from build123d import *

# Parameters (mm, degrees)
SKETCH1_W           = 6
SKETCH1_H           = 10
BOSS_EXTRUDE1_DEPTH = 8
FILLET2_RADIUS      = 3
FILLET2_LENGTH      = 10
SKETCH2_R           = 1.5
BOSS_EXTRUDE2_DEPTH = 2


with BuildPart() as part:
    # Sketch1 → Boss-Extrude1 (new body)
    with BuildSketch(Plane.XY):
        Rectangle(SKETCH1_W, SKETCH1_H)
    extrude(amount=BOSS_EXTRUDE1_DEPTH)

    # Fillet2: full round fillet: the end face becomes a half cylinder, R = half its width
    fillet2_face = Plane((0, 0, 8), x_dir=(0, -1, 0), z_dir=(0, 0, 1))  # on the end face: x along it, z out of the body
    fillet2_slab = fillet2_face.offset(-FILLET2_RADIUS / 2) * Box(FILLET2_LENGTH, 2 * FILLET2_RADIUS, FILLET2_RADIUS, mode=Mode.PRIVATE)  # the body's end, R deep
    fillet2_round = Plane((0, 0, 5), x_dir=(0, 0, 1), z_dir=(0, -1, 0)) * Cylinder(FILLET2_RADIUS, FILLET2_LENGTH, mode=Mode.PRIVATE)  # its axis R under the face
    add(fillet2_slab - fillet2_round, mode=Mode.SUBTRACT)

    # Sketch2 → Boss-Extrude2 (add)
    with BuildSketch(Plane(origin=(0, 5, 0), x_dir=(1, 0, 0), z_dir=(0, 1, 0))):
        with Locations(Location((0, -5, 0), (0, 0, 90))):
            Circle(SKETCH2_R)
    extrude(amount=BOSS_EXTRUDE2_DEPTH)


solid = part.part
Model file for the job. Use its own axes, mm. A direction names the side the tool comes from. Coordinates: 2 decimals unless noted, no trailing zeros. Loops run counter-clockwise (first coordinate to the right, second up) from the corner with the lowest first, then second, coordinate; pieces in that order, holes last. Notation, with made-up numbers: (70.5, -18.75) -> (127.5, -18.75) arc R28 ccw to (127.5, 17.25) -> close; hole circle Ø6 at (50.5, 74). An arc over 180 degrees is marked (long way). Use one line per item in the form item = value. Start each with the question number.
(1) Probe probe 1 along Y at (x, z) = (0.7, 0.5); probe 2 along X at (y, z) = (5.5, 5); probe 3 along Z at (x, y) = (-1.65, 2.5). List the from-to ranges inside material, lowest first. Write a range as from..to.
(2) Cut at B-B on y = -1. Give the cut face in (x, z).
(3) Cut at D-D on y = 6.25. Give the cut face in (x, z), and give its area (3 significant figures).
(4) Tool access for faces 1 (the flat face through (0, -5, 4)), 2 (the cylindrical face through (-0.07, 5.99, 6.5)): list every direction of +Z, -Z, +X, -X, +Y, -Y with a clear straight run to the whole face (end or side of a thin tool).
(5) Cut at C-C on z = 5.25. Give the cut face in (x, y), and give its area (3 significant figures).
(6) Cut at A-A on x = 0. Give the cut face in (y, z), and give its area (3 significant figures).
Values:
q1.probe_1 = -5..5
q1.probe_2 = -1.5..1.5
q1.probe_3 = 0..7.51
q2.outline = (-3, 0) -> (3, 0) -> (3, 5) arc R3 ccw to (-3, 5) -> close
q3.outline = circle Ø3 at (0, 5)
q3.area = 7.07 mm2
q4.face_1 = +Z, -Z, +X, -X, -Y
q4.face_2 = +Y
q5.outline = (-2.99, -5) -> (2.99, -5) -> (2.99, 5) -> (1.48, 5) -> (1.48, 7) -> (-1.48, 7) -> (-1.48, 5) -> (-2.99, 5) -> close
q5.area = 65.7 mm2
q6.outline = (-5, 0) -> (5, 0) -> (5, 3.5) -> (7, 3.5) -> (7, 6.5) -> (5, 6.5) -> (5, 8) -> (-5, 8) -> close
q6.area = 86.0 mm2
